Input: part model. Units: mm. Frame: model coordinates. A direction names the side the tool comes from. Round coordinates to 2 decimals unless told otherwise and drop trailing zeros. Loops run counter-clockwise (first coordinate to the right, second up) from the corner with the lowest first, then second, coordinate; pieces in that order, holes last. Notation, with made-up numbers: (74.5, 1.5) -> (130.5, 1.5) arc R25 ccw to (130.5, 16.5) -> close; hole circle Ø6 at (-34, 27.5). An arc over 180 degrees is marked (long way). Answer as a JSON object with one key per item and string values. Group by question number.
Item 1: Section query D-D on x = 3.81. Return loops of the section in (y, z).
Item 2: Section query B-B on y = 4.5. Count the separate pieces of the cut face and the enclosed holes in it, and give its area (3 significant figures).
Item 3: Draft query along Z for faces 1 (the flat face through (19, 4, 0)), 2 (the flat face through (34, 2.87, -5)), 3 (the flat face through (19, 0, -5)). Return one class per face: released by +Z, released by -Z, zero draft, split by the parting line, or undercut.
Item 4: Material intervals for line 1 (Z direction, x = 34.29, y = 5.4); line 2 (X direction, y = 3, z = -5.5); line 3 (X direction, y = 7, z = -5.75), sorted ascending. Write a range as [from, to].
Item 5: Section query C-C on z = -5.75. Return loops of the section in (x, y).
Item 6: Set-up query: faces 4 (the flat face through (19, 4, -10.16)), 5 (the flat face through (11, 2.87, -5)). Return all of +Z, -Z, +X, -X, +Y, -Y with unobstructed straight access to the full face (end or side cutting, diameter ignored); none if empty.
Item 7: Section query A-A on x = 11.43. Return loops of the section in (y, z).
Item 8: Pin query (flat end, axial travel): pin 1 (1 mm diameter, centred on x = 33.5, z = -5, fed in from +Y). Return the tip coordinate at first contact, or that it passes through.
from build123d import *

# Parameters (mm, degrees)
SKETCH3_W           = 38.1
SKETCH3_H           = 10.16
BOSS_EXTRUDE2_DEPTH = 7.62
CUT_EXTRUDE1_START  = 7.62
SKETCH1_R           = 1.5748
SKETCH1_R_2         = 1.5875
SKETCH1_R_3         = 1.6002
SKETCH1_R_4         = 1.6129
SKETCH1_R_5         = 1.6256
CUT_EXTRUDE1_DEPTH  = 4.7498


with BuildPart() as part:
    # Sketch3 → Boss-Extrude2 (new body)
    with BuildSketch(Plane(origin=(0, 0, 0), x_dir=(1, 0, 0), z_dir=(0, 1, 0))):
        with Locations((19.05, 5.08)):
            Rectangle(SKETCH3_W, SKETCH3_H)
    extrude(amount=BOSS_EXTRUDE2_DEPTH)

    # Sketch1 → Cut-Extrude1 (cut)
    with BuildSketch(Plane(origin=(0, 0, 0), x_dir=(1, 0, 0), z_dir=(0, 1, 0)).offset(CUT_EXTRUDE1_START)):
        with Locations(Location((3.81, 4.807346471, 0), (0, 0, 90))):
            Circle(SKETCH1_R)
        with Locations(Location((11.43, 4.807346471, 0), (0, 0, 90))):
            Circle(SKETCH1_R_2)
        with Locations(Location((19.05, 4.807346471, 0), (0, 0, 90))):
            Circle(SKETCH1_R_3)
        with Locations(Location((26.67, 4.807346471, 0), (0, 0, 90))):
            Circle(SKETCH1_R_4)
        with Locations(Location((34.29, 4.807346471, 0), (0, 0, 90))):
            Circle(SKETCH1_R_5)
    extrude(amount=-CUT_EXTRUDE1_DEPTH, mode=Mode.SUBTRACT)


solid = part.part
Solved:
{
 "1": {"outline": "(0, -10.16) -> (7.62, -10.16) -> (7.62, -6.38) -> (2.87, -6.38) -> (2.87, -3.23) -> (7.62, -3.23) -> (7.62, 0) -> (0, 0) -> close"},
 "2": {"separate pieces": "1", "enclosed holes": "5", "area": "347 mm²"},
 "3": {"face 1": "released by +Z", "face 2": "undercut", "face 3": "zero draft"},
 "4": {"line 1": "[-10.16, -6.43], [-3.18, 0]", "line 2": "[0, 2.4], [5.22, 10], [12.86, 17.61], [20.49, 25.21], [28.13, 32.82], [35.76, 38.1]", "line 3": "[0, 2.55], [5.07, 10.15], [12.71, 17.76], [20.34, 25.36], [27.98, 32.97], [35.61, 38.1]"},
 "5": {"outline": "(0, 0) -> (38.1, 0) -> (38.1, 7.62) -> (35.61, 7.62) -> (35.61, 2.87) -> (32.97, 2.87) -> (32.97, 7.62) -> (27.98, 7.62) -> (27.98, 2.87) -> (25.36, 2.87) -> (25.36, 7.62) -> (20.34, 7.62) -> (20.34, 2.87) -> (17.76, 2.87) -> (17.76, 7.62) -> (12.71, 7.62) -> (12.71, 2.87) -> (10.15, 2.87) -> (10.15, 7.62) -> (5.07, 7.62) -> (5.07, 2.87) -> (2.55, 2.87) -> (2.55, 7.62) -> (0, 7.62) -> close"},
 "6": {"face 4": "-Z, +X, -X, +Y, -Y", "face 5": "+Y"},
 "7": {"outline": "(0, -10.16) -> (7.62, -10.16) -> (7.62, -6.39) -> (2.87, -6.39) -> (2.87, -3.22) -> (7.62, -3.22) -> (7.62, 0) -> (0, 0) -> close"},
 "8": {"pin 1": "y = 2.87"}
}
